from build123d import *

# Parameters (mm, degrees)
SKETCH1_W           = 30
SKETCH1_H           = 60
BOSS_EXTRUDE1_DEPTH = 457
SKETCH2_W           = 10
SKETCH2_H           = 8.5
CUT_EXTRUDE1_DEPTH  = 500
SKETCH3_W           = 10
SKETCH3_H           = 8.5
CUT_EXTRUDE2_DEPTH  = 42.89


with BuildPart() as part:
    # Sketch1 → Boss-Extrude1 (new body)
    with BuildSketch(Plane.XY):
        with Locations((15, 30)):
            Rectangle(SKETCH1_W, SKETCH1_H)
    extrude(amount=BOSS_EXTRUDE1_DEPTH)

    # Sketch2 → Cut-Extrude1 (cut)
    with BuildSketch(Plane.XY.offset(457)):
        with Locations((5, 38.75)):
            Rectangle(SKETCH2_W, SKETCH2_H)
        with Locations((5, 55.75)):
            Rectangle(SKETCH2_W, SKETCH2_H)
    extrude(amount=-CUT_EXTRUDE1_DEPTH, mode=Mode.SUBTRACT)

    # Sketch3 → Cut-Extrude2 (cut)
    with BuildSketch(Plane(origin=(0, 0, 0), x_dir=(-1, 0, 0), z_dir=(0, 0, -1))):
        with Locations((-5, 21.75)):
            Rectangle(SKETCH3_W, SKETCH3_H)
    extrude(amount=-CUT_EXTRUDE2_DEPTH, mode=Mode.SUBTRACT)


solid = part.part
The listing builds one solid part. Answer for the finished solid, in the listing's coordinates (mm). A direction names the side the tool comes from. Give positions to 0.01 mm unless a question says otherwise; leave off trailing zeros. Write each loop counter-clockwise with the first axis right and the second up, starting at its lowest first coordinate (ties: lowest second). Pieces come first, ordered by that corner, then holes. Notation, with made-up numbers: (59, -27) - (75, -27) arc R12 cw to (75, -10) - close; hole circle Ø11 at (-16, 46.25). An arc over 180 degrees is marked (long way). Use a Markdown table: item, result.
1. Find the intervals of material crossed by probe 1 along Y at (x, z) = (4.25, 147.5); probe 2 along Z at (x, y) = (6, 22.5); probe 3 along X at (y, z) = (55, 179.5), in increasing order. Write a range as from..to.
Values follow:
| item | result |
|---|---|
| probe 1 | y = 0..34.5, 43..51.5 |
| probe 2 | z = 42.89..457 |
| probe 3 | x = 10..30 |
2. Section A-A on x = 5.25 is taken. Write down the section's boundary in (y, z).
Values follow:
| item | result |
|---|---|
| outline | (0, 0) - (17.5, 0) - (17.5, 42.89) - (26, 42.89) - (26, 0) - (34.5, 0) - (34.5, 457) - (0, 457) - close; (43, 0) - (51.5, 0) - (51.5, 457) - (43, 457) - close |
3. Section B-B on z = 224 is taken. Write down the section's boundary in (x, y).
Values follow:
| item | result |
|---|---|
| outline | (0, 0) - (30, 0) - (30, 60) - (10, 60) - (10, 51.5) - (0, 51.5) - (0, 43) - (10, 43) - (10, 34.5) - (0, 34.5) - close |
4. For a pull along Y with two mould halves and no side action, classify faces 5 (the flat face through (20, 60, 225)), 6 (the flat face through (5, 34.5, 232)), 7 (the flat face through (15, 30, 0)) as released by +Y, released by -Y, zero draft, split by the parting line, or undercut.
Values follow:
| item | result |
|---|---|
| face 5 | released by +Y |
| face 6 | undercut |
| face 7 | zero draft |
5. A tool of negligible diameter and unlimited length cuts with its end or side. For faces 1 (the flat face through (10, 39, 232)), 2 (the flat face through (5, 26, 21)), 3 (the flat face through (10, 56, 232)), 4 (the flat face through (30, 30, 225)), from which of +Z, -Z, +X, -X, +Y, -Y can it reach the whole face along a straight path? Write none if from no direction.
Values follow:
| item | result |
|---|---|
| face 1 | +Z, -Z, -X |
| face 2 | -Z, -X |
| face 3 | +Z, -Z, -X, +Y |
| face 4 | +Z, -Z, +X, +Y, -Y |
6. Each of these flat-tipped pins is pushed along its axis until it touches: P1, Ø9.5, axis at y = 57, z = 126, coming from the -X side; P2, Ø3, axis at x = 6.5, z = 14.5, coming from the +Y side. Where does it stop, or does it pass through?
Values follow:
| item | result |
|---|---|
| P1 | stops at x = 10 |
| P2 | stops at y = 51.5 |
